Verification items for this drawing (mm, ordinates from the low corner). A direction names the side the tool comes from. Round coordinates to 2 decimals unless told otherwise and drop trailing zeros. Loops run counter-clockwise (first coordinate to the right, second up) from the corner with the lowest first, then second, coordinate; pieces in that order, holes last. Notation, with made-up numbers: (6, 25) - (52, 25) arc R37 ccw to (52, 62) - close; hole circle Ø1 at (41, 69.25). An arc over 180 degrees is marked (long way). Put each result on its own line as item: value.
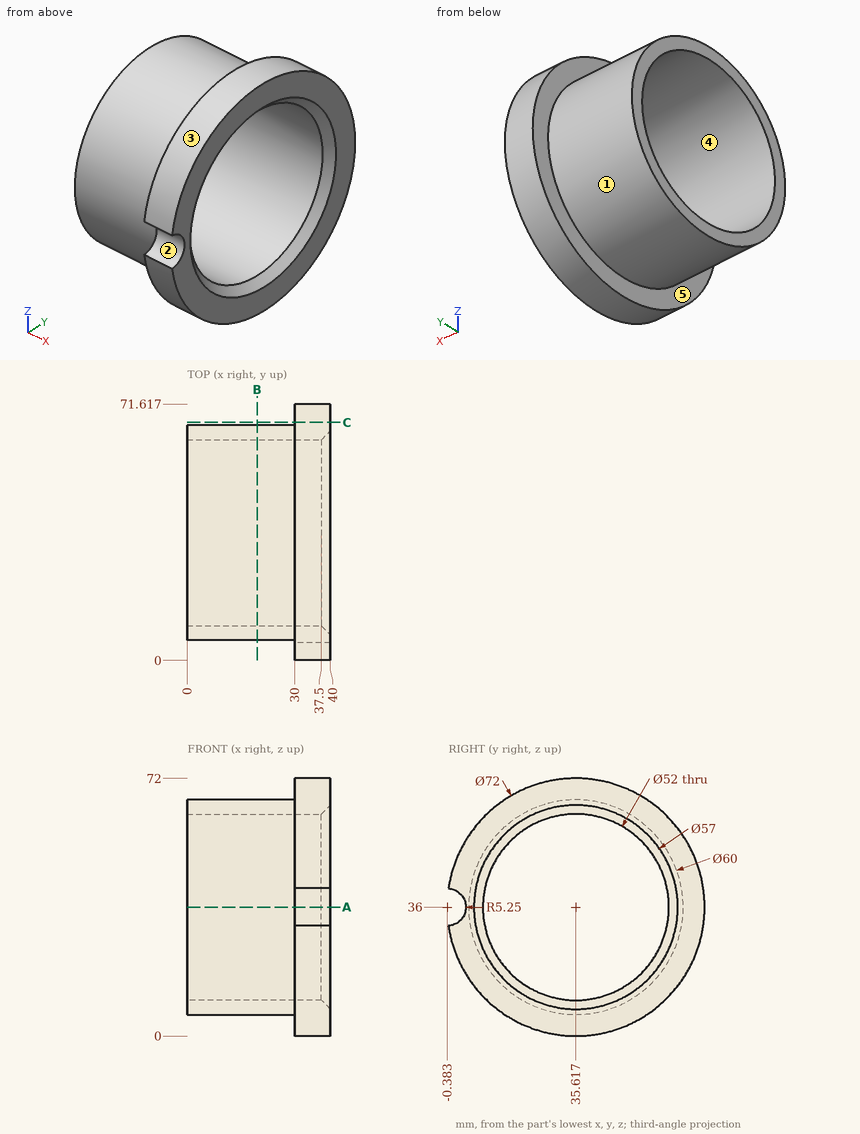
Item 1: Go/stop test with flat-tipped pins: pin 1 (4 mm diameter, centred on x = 11.5, y = 46.5, fed in from +Z) (1 decimal); pin 2 (1.5 mm diameter, centred on x = 6.5, y = 32, fed in from +Z); pin 3 (3 mm diameter, centred on x = 31, y = 17, fed in from -Z). Record where each tip stops, or that it passes through.
Filled sheet:
pin 1: z = 64.7
pin 2: z = 65.86
pin 3: z = 4.33
Item 2: Section check B-B on x = 19.5. Enter the section's corners in (y, z), then the cut area to 3 significant figures.
Filled sheet:
outline: circle Ø60 at (35.62, 36); hole circle Ø52 at (35.62, 36)
area: 704 mm²
Item 3: Tool access check on the marked faces 1 and 2. Record the directions out of +Z, -Z, +X, -X, +Y, -Y that give a thin tool (end or side, any length) a straight path to the whole face; none if there is none.
Filled sheet:
face 1: -X
face 2: +X, -X, -Y
Item 4: Section check C-C on y = 66.5. Enter the section's corners in (x, z), then the cut area to 3 significant figures.
Filled sheet:
outline: (30, 17.5) - (40, 17.5) - (40, 54.5) - (30, 54.5) - close
area: 370 mm²
Item 5: Release check for a two-part mould opening along Y. For the marked faces 3, 4 and 5 record: +Y half, -Y half, draft (parallel to the pull), parting line (faces both ways), or undercut.
Filled sheet:
face 3: parting line
face 4: undercut
face 5: draft
Item 6: Section check A-A on z = 36. Enter the section's corners in (x, y).
Filled sheet:
outline: (0, 5.62) - (30, 5.62) - (30, 4.87) - (40, 4.87) - (40, 7.12) - (37.5, 9.62) - (0, 9.62) - close; (0, 61.62) - (37.5, 61.62) - (40, 64.12) - (40, 71.62) - (30, 71.62) - (30, 65.62) - (0, 65.62) - close
Item 7: Thickness scan on line 1 (Y direction, x = 15, z = 36); line 2 (Y direction, x = 8.5, z = 32) (1 decimal); line 3 (Z direction, x = 6.5, y = 50). Record the ranges inside material, lowest first. Write a range as from..to.
Filled sheet:
line 1: 5.62..9.62, 61.62..65.62
line 2: 5.9..9.9, 61.3..65.3
line 3: 9.67..14.34, 57.66..62.33
